Geometry: see drawing. Coordinates: mm, zero at the bounding-box minimum. Coordinates: 2 decimals unless noted, no trailing zeros. Order: outer loops, then holes, each group sorted by start corner. A loop starts at its lowest first (then second) coordinate and runs counter-clockwise, first axis right, second up.
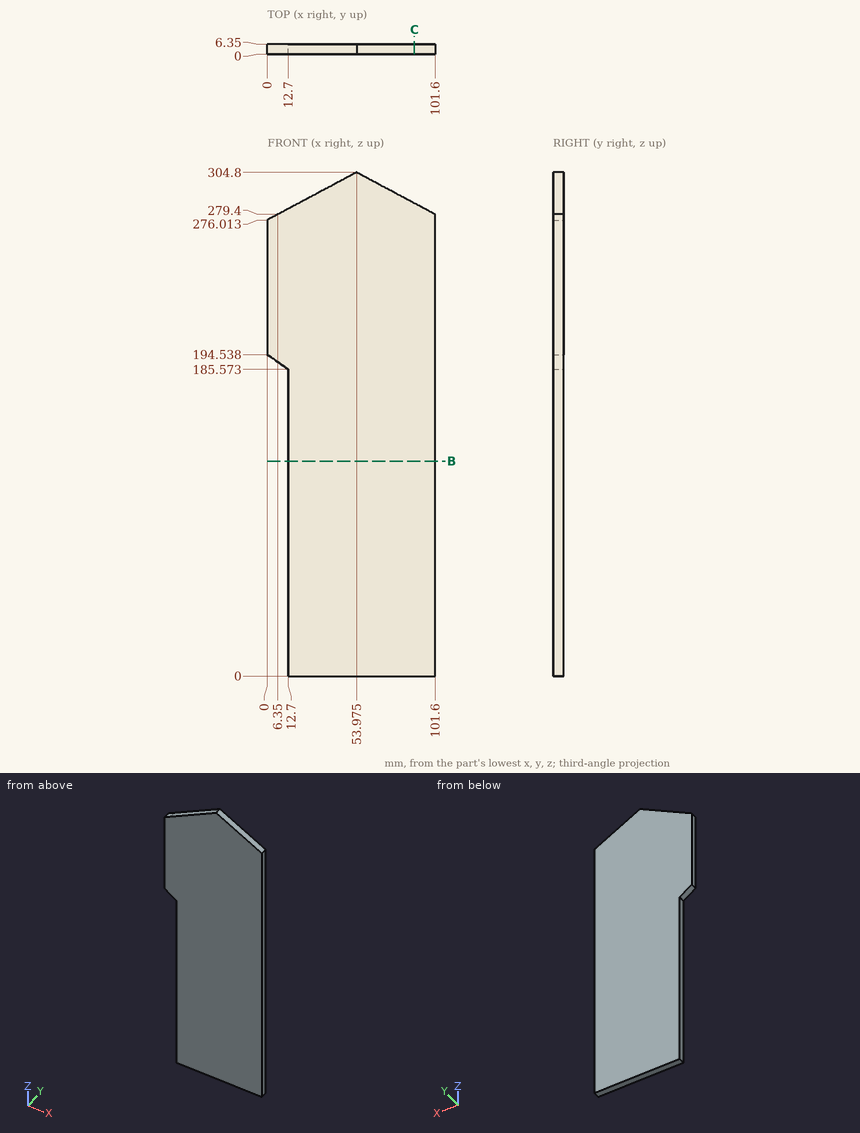
Q1. Pin query (flat end, axial travel): P1, Ø1, axis at x = 63.5, y = 3, coming from the +Z side; P2, Ø3, axis at y = 2.5, z = 51.5, coming from the -X side; P3, Ø1, axis at x = 69.5, y = 1.5, coming from the +Z side. Return the tip coordinate at first contact, or that it passes through.
Solutions:
P1: stops at z = 299.99
P2: stops at x = 12.7
P3: stops at z = 296.79
Q2. Material intervals for line 1 along X through (y, z) = (5.25, 119); line 2 along Z through (x, y) = (69.5, 2); line 3 along Z through (x, y) = (79, 3), sorted ascending.
Solutions:
line 1: x = 12.7 to 101.6
line 2: z = 0 to 296.52
line 3: z = 0 to 291.45
Q3. Section query C-C on x = 89. Output: boundary loops of the cut face in (y, z), plus the area to 3 significant figures.
Solutions:
outline: (0, 0) - (6.35, 0) - (6.35, 286.12) - (0, 286.12) - close
area: 1,820 mm2
Q4. Section query B-B on z = 130. Output: boundary loops of the cut face in (x, y).
Solutions:
outline: (12.7, 0) - (101.6, 0) - (101.6, 6.35) - (12.7, 6.35) - close
